```python
from build123d import *

# Parameters (mm, degrees)
CROQUIS1_W              = 50
CROQUIS1_H              = 70
SALIENTE_EXTRUIR1_DEPTH = 1
CROQUIS1_3_W            = 52
CROQUIS1_3_H            = 72
CROQUIS1_3_W_2          = 50
CROQUIS1_3_H_2          = 70
SALIENTE_EXTRUIR2_DEPTH = 21
CROQUIS3_W              = 5
CROQUIS3_H              = 6
CORTAR_EXTRUIR1_DEPTH   = 21
CROQUIS4_W              = 10
CROQUIS4_H              = 2.5
CORTAR_EXTRUIR3_DEPTH   = 29
CROQUIS5_W              = 10
CROQUIS5_H              = 5
CORTAR_EXTRUIR4_DEPTH   = 29


with BuildPart() as part:
    # Croquis1 → Saliente-Extruir1 (new body)
    with BuildSketch(Plane(origin=(0, 0, 0), x_dir=(1, 0, 0), z_dir=(0, 1, 0))):
        with Locations((25, 35)):
            Rectangle(CROQUIS1_W, CROQUIS1_H)
    extrude(amount=SALIENTE_EXTRUIR1_DEPTH)

    # Croquis1_3 → Saliente-Extruir2 (add)
    with BuildSketch(Plane(origin=(0, 0, 0), x_dir=(1, 0, 0), z_dir=(0, 1, 0))):
        with Locations((25, 35)):
            Rectangle(CROQUIS1_3_W, CROQUIS1_3_H)
        with Locations((25, 35)):
            Rectangle(CROQUIS1_3_W_2, CROQUIS1_3_H_2, mode=Mode.SUBTRACT)
    extrude(amount=SALIENTE_EXTRUIR2_DEPTH)

    # Croquis3 → Cortar-Extruir1 (cut)
    with BuildSketch(Plane(origin=(0, 0, -71), x_dir=(-1, 0, 0), z_dir=(0, 0, -1))):
        with Locations((-27.5, 12.33)):
            Rectangle(CROQUIS3_W, CROQUIS3_H)
        with Locations((-22.5, 12.33)):
            Rectangle(CROQUIS3_W, CROQUIS3_H)
    extrude(amount=-CORTAR_EXTRUIR1_DEPTH, mode=Mode.SUBTRACT)

    # Croquis4 → Cortar-Extruir3 (cut)
    with BuildSketch(Plane(origin=(51, 0, 0), x_dir=(0, 0, -1), z_dir=(1, 0, 0))):
        with Locations((25, 9.25)):
            Rectangle(CROQUIS4_W, CROQUIS4_H)
        with Locations((25, 11.75)):
            Rectangle(CROQUIS4_W, CROQUIS4_H)
        with Locations((54, 9.25)):
            Rectangle(CROQUIS4_W, CROQUIS4_H)
        with Locations((54, 11.75)):
            Rectangle(CROQUIS4_W, CROQUIS4_H)
    extrude(amount=-CORTAR_EXTRUIR3_DEPTH, mode=Mode.SUBTRACT)

    # Croquis5 → Cortar-Extruir4 (cut)
    with BuildSketch(Plane.ZY.offset(1)):
        with Locations((-57, 10.5)):
            Rectangle(CROQUIS5_W, CROQUIS5_H)
    extrude(amount=-CORTAR_EXTRUIR4_DEPTH, mode=Mode.SUBTRACT)


solid = part.part
```
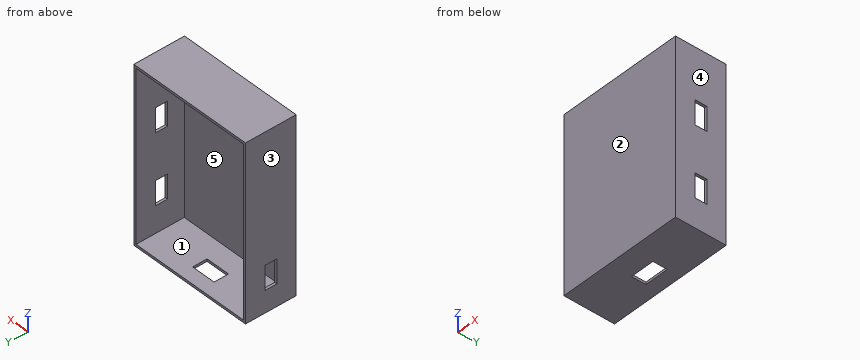
Part model, mm, in its own coordinate system. Face numbers are marked on the shaded views. A direction names the side the tool comes from. Give positions to 0.01 mm unless a question says otherwise; leave off trailing zeros. Order: outer loops, then holes, each group sorted by start corner. A loop starts at its lowest first (then second) coordinate and runs counter-clockwise, first axis right, second up. Notation, with made-up numbers: M 36,15 L 59,15 A27 cw 59,45 Z; hole C -22,34.5 d7. An arc over 180 degrees is marked long. Use a Markdown table: item, result. Add a question column.
(1) 3-axis set-ups, long thin cutter, end or side, ignore diameter. For the marked faces 4 and 5: which of +Z, -Z, +X, -X, +Y, -Y reach the whole face in a straight line?
(2) Mould opens along X. For the marked faces 1, 2 and 3 say: +X half, -X half, draft (parallel to the pull), parting line (faces both ways), or undercut.
(3) Saw through at A-A, the plane x = 24. Give the cut face in (y, z).
(4) Saw through at C-C, the plane z = -25.5. Give the cut face in (x, y), and give its area (3 significant figures).
(5) Drop a flat-ended pin along its axis: P1, Ø1, axis at x = 41.5, z = -16.5, coming from the +Y side. Give the stop position or say it passes through.
(6) Saw through at D-D, the plane y = 4. Give the cut face in (x, z), and give its area (3 significant figures).
(7) Probe line 1 along X through (y, z) = (15.75, -66.5); line 2 along Z through (x, y) = (22.5, 7.25); line 3 along Y through (x, z) = (23.5, -61). List the from-to ranges inside material, lowest first. Write a range as [from, to].
(8) Saw through at B-B, the plane z = -56. Give the cut face in (x, y).
Answer key:
| question | item | result |
|---|---|---|
| 1 | face 4 | +Z, -Z, +X, +Y, -Y |
| 1 | face 5 | +Y |
| 2 | face 1 | undercut |
| 2 | face 2 | draft |
| 2 | face 3 | -X half |
| 3 | outline | M 0,-71 L 9.33,-71 L 9.33,-70 L 1,-70 L 1,0 L 21,0 L 21,1 L 0,1 Z; M 15.33,-71 L 21,-71 L 21,-70 L 15.33,-70 Z |
| 4 | outline | M -1,0 L 51,0 L 51,8 L 50,8 L 50,1 L 0,1 L 0,21 L -1,21 Z; M 50,13 L 51,13 L 51,21 L 50,21 Z |
| 4 | area | 87.0 mm^2 |
| 5 | P1 | y = 1 |
| 6 | outline | M -1,-71 L 51,-71 L 51,1 L -1,1 Z; hole M 0,-70 L 50,-70 L 50,0 L 0,0 Z |
| 6 | area | 244 mm^2 |
| 7 | line 1 | [-1, 0], [50, 51] |
| 7 | line 2 | [-71, -70], [0, 1] |
| 7 | line 3 | [0, 1] |
| 8 | outline | M -1,0 L 51,0 L 51,8 L 50,8 L 50,1 L 0,1 L 0,8 L -1,8 Z; M -1,13 L 0,13 L 0,21 L -1,21 Z; M 50,13 L 51,13 L 51,21 L 50,21 Z |
